Check sheet for the drawn part. Datum: minimum x, y, z corner. Units: mm. Give positions to 0.01 mm unless a question says otherwise; leave off trailing zeros. Write each loop counter-clockwise with the first axis right and the second up, starting at its lowest first coordinate (ties: lowest second). Pieces come first, ordered by that corner, then holes. Notation, with made-up numbers: (49.25, 1.25) -> (63.25, 1.25) arc R20 cw to (63.25, 33.25) -> close; hole circle Ø5 at (9.5, 37.5). An arc over 180 degrees is marked (long way). Write item = value, one per line. Start each with the question number.
1. Depth check by flat-ended pin: P1, Ø2, axis at y = 4, z = 120, coming from the -X side; P2, Ø9.5, axis at x = 108.6, z = 30, coming from the +Y side. Enter the tip coordinate at first touch or a pass-through.
2. Cross-section at C-C, the plane y = 4.5. Record the cut outline in (x, z).
3. Cross-section at B-B, the plane x = 108.6. Record the cut outline in (y, z).
4. Cross-section at A-A, the plane z = 30. Record the cut outline in (x, y).
5. Cross-section at D-D, the plane x = 32. Record the cut outline in (y, z).
6. Thickness scan on line 1 along Z through (x, y) = (108.6, 4.5); line 2 along Z through (x, y) = (6, 2); line 3 along X through (y, z) = (6.25, 32). Record the ranges inside material, lowest first.
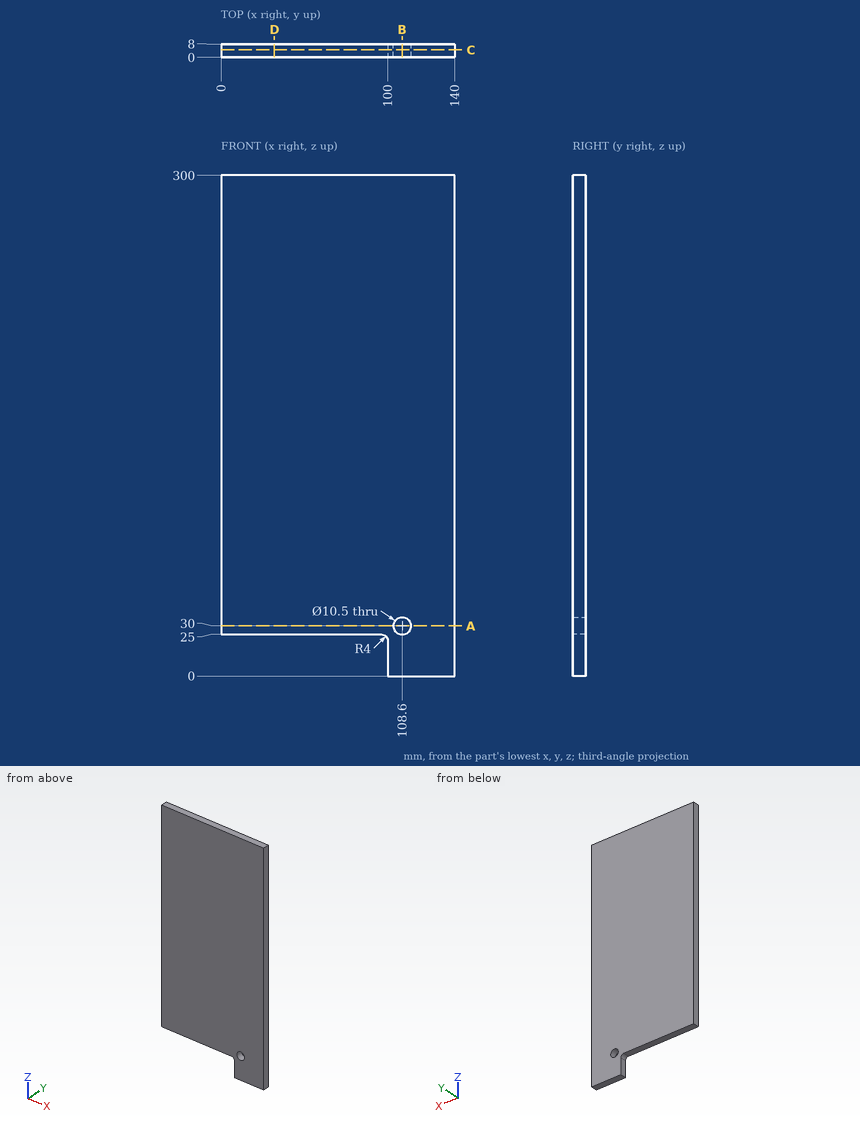
Answers:
q1.P1 = 0
q1.P2 = through
q2.outline = (0, 25) -> (96, 25) arc R4 cw to (100, 21) -> (100, 0) -> (140, 0) -> (140, 300) -> (0, 300) -> close; hole circle Ø10.5 at (108.6, 30)
q3.outline = (0, 0) -> (8, 0) -> (8, 24.75) -> (0, 24.75) -> close; (0, 35.25) -> (8, 35.25) -> (8, 300) -> (0, 300) -> close
q4.outline = (0, 0) -> (103.35, 0) -> (103.35, 8) -> (0, 8) -> close; (113.85, 0) -> (140, 0) -> (140, 8) -> (113.85, 8) -> close
q5.outline = (0, 25) -> (8, 25) -> (8, 300) -> (0, 300) -> close
q6.line_1 = 0 to 24.75, 35.25 to 300
q6.line_2 = 25 to 300
q6.line_3 = 0 to 103.75, 113.45 to 140
